Verification items for this drawing (mm, ordinates from the low corner). Coordinates: 2 decimals unless noted, no trailing zeros. Write each loop counter-clockwise with the first axis right and the second up, starting at its lowest first coordinate (ties: lowest second). Pieces come first, ordered by that corner, then holes.
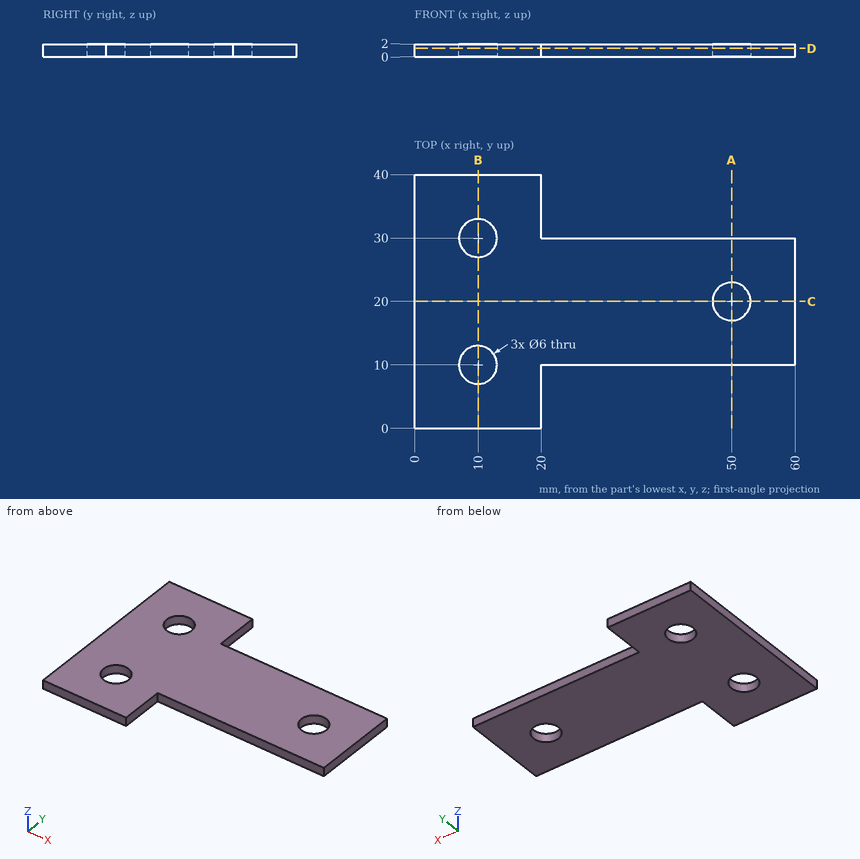
1. Gauge pin test, flat ends, axial feed: pin 1 Ø0.6 at (y, z) = (4.5, 1.5) entering from +X; pin 2 Ø1 at (x, z) = (46.5, 1.5) entering from +Y. Record the tip position at first contact, or that the pin passes through.
Computed values:
pin 1: stops at x = 20
pin 2: stops at y = 30
2. Sectioned sample at A-A, the plane x = 50. Record the boundary of the cut face in (y, z).
Computed values:
outline: (10, 0) - (17, 0) - (17, 2) - (10, 2) - close; (23, 0) - (30, 0) - (30, 2) - (23, 2) - close
3. Thickness scan on line 1 along Y through (x, z) = (10, 1.1); line 2 along X through (y, z) = (33.5, 1.5); line 3 along Y through (x, z) = (49, 0.3). Record the ranges inside material, lowest first.
Computed values:
line 1: y = 0 to 7, 13 to 27, 33 to 40
line 2: x = 0 to 20
line 3: y = 10 to 17.17, 22.83 to 30
4. Sectioned sample at B-B, the plane x = 10. Record the boundary of the cut face in (y, z).
Computed values:
outline: (0, 0) - (7, 0) - (7, 2) - (0, 2) - close; (13, 0) - (27, 0) - (27, 2) - (13, 2) - close; (33, 0) - (40, 0) - (40, 2) - (33, 2) - close
5. Sectioned sample at C-C, the plane y = 20. Record the boundary of the cut face in (x, z), and give its area (3 significant figures).
Computed values:
outline: (0, 0) - (47, 0) - (47, 2) - (0, 2) - close; (53, 0) - (60, 0) - (60, 2) - (53, 2) - close
area: 108 mm2
6. Sectioned sample at D-D, the plane z = 1.3. Record the boundary of the cut face in (x, y).
Computed values:
outline: (0, 0) - (20, 0) - (20, 10) - (60, 10) - (60, 30) - (20, 30) - (20, 40) - (0, 40) - close; hole circle Ø6 at (10, 10); hole circle Ø6 at (10, 30); hole circle Ø6 at (50, 20)
